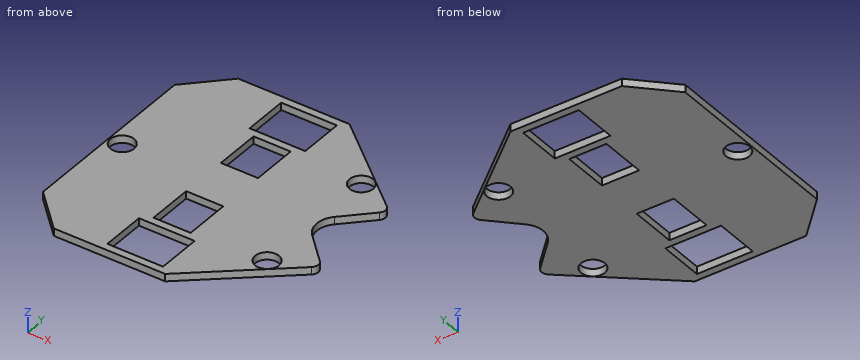
```python
from build123d import *

# Parameters (mm, degrees)
SKETCH_R      = 16
SKETCH_W      = 75
SKETCH_H      = 60
SKETCH_W_2    = 50
SKETCH_H_2    = 62
EXTRUDE_DEPTH = 10


with BuildPart() as part:
    # Sketch → Extrude (new body)
    with BuildSketch(Plane.XY):
        with BuildLine():
            Line((-152.5, 125), (-152.5, -125))
            Line((-152.5, -125), (-102.5, -175))
            Line((-102.5, -175), (47.5, -175))
            Line((47.5, -175), (171.038135, -71.339197))
            ThreePointArc((171.038135, -71.339197), (174.600715, -64.114951), (171.6813, -56.607707))
            Line((136.286797, -21.213204), (171.6813, -56.607707))
            ThreePointArc((136.286797, 21.213204), (127.5, 0), (136.286797, -21.213204))
            Line((171.6813, 56.607707), (136.286797, 21.213204))
            ThreePointArc((171.6813, 56.607707), (174.600715, 64.114951), (171.038135, 71.339197))
            Line((171.038135, 71.339197), (47.5, 175))
            Line((47.5, 175), (-102.5, 175))
            Line((-102.5, 175), (-152.5, 125))
        make_face()
        with Locations((124, 89.5)):
            Circle(SKETCH_R, mode=Mode.SUBTRACT)
        with Locations((124, -89.5)):
            Circle(SKETCH_R, mode=Mode.SUBTRACT)
        with Locations((-134.5, 0)):
            Circle(SKETCH_R, mode=Mode.SUBTRACT)
        with Locations((0, 135)):
            Rectangle(SKETCH_W, SKETCH_H, mode=Mode.SUBTRACT)
        with Locations((0, -135)):
            Rectangle(SKETCH_W, SKETCH_H, mode=Mode.SUBTRACT)
        with Locations((0, 64)):
            Rectangle(SKETCH_W_2, SKETCH_H_2, mode=Mode.SUBTRACT)
        with Locations((0, -64)):
            Rectangle(SKETCH_W_2, SKETCH_H_2, mode=Mode.SUBTRACT)
    extrude(amount=EXTRUDE_DEPTH)


with BuildPart() as part_1:
    # Extrude placement: moved
    add(part.part.moved(Location((0, 0, -30))))


solid = part_1.part
```
The listing builds one solid part. Answer for the finished solid, in the listing's coordinates (mm). Coordinates: 2 decimals unless noted, no trailing zeros. Loops run counter-clockwise (first coordinate to the right, second up) from the corner with the lowest first, then second, coordinate; pieces in that order, holes last. Notation, with made-up numbers: (51.5, 80.5) -> (102.5, 80.5) arc R20 cw to (102.5, 110.5) -> close; hole circle Ø10 at (82.5, 48). An arc over 180 degrees is marked (long way). Return JSON: item names as keys, results as strings. Group by question number.
(1) A cutting plane is placed at B-B on x = -134.5. Write down the section's boundary in (y, z), and give its area (3 significant figures).
(2) Given pin 1 Ø3 at (y, z) = (129.5, -23.5) entering from +X; pin 2 Ø3 at (x, z) = (109.5, -29) entering from +Y; pin 3 Ø2 at (x, z) = (91.5, -24.5) entering from -Y, each flat-ended and moving along its own axis, determine where each tip first touches the part or whether it passes through.
(3) A cutting plane is placed at A-A on z = -25. Count the separate pieces of the cut face and the enclosed holes in it, and give its area (3 significant figures).
(4) A cutting plane is placed at D-D on x = 32. Write down the section's boundary in (y, z).
(5) A cutting plane is placed at C-C on y = 0. Write down the section's boundary in (x, z), and give its area (3 significant figures).
(6) Find the intervals of material crossed by probe 1 along Y at (x, z) = (17.5, -26); probe 2 along Y at (x, z) = (130, -27.5); probe 3 along Y at (x, z) = (124, -23), in increasing order. Write a range as from..to.
The answers:
{
 "1": {"outline": "(-143, -30) -> (-16, -30) -> (-16, -20) -> (-143, -20) -> close; (16, -30) -> (143, -30) -> (143, -20) -> (16, -20) -> close", "area": "2,540 mm^2"},
 "2": {"pin 1": "stops at x = 103.51", "pin 2": "stops at y = 124.23", "pin 3": "stops at y = -138.92"},
 "3": {"separate pieces": "1", "enclosed holes": "7", "area": "77,500 mm^2"},
 "4": {"outline": "(-175, -30) -> (-165, -30) -> (-165, -20) -> (-175, -20) -> close; (-105, -30) -> (105, -30) -> (105, -20) -> (-105, -20) -> close; (165, -30) -> (175, -30) -> (175, -20) -> (165, -20) -> close"},
 "5": {"outline": "(-152.5, -30) -> (-150.5, -30) -> (-150.5, -20) -> (-152.5, -20) -> close; (-118.5, -30) -> (127.5, -30) -> (127.5, -20) -> (-118.5, -20) -> close", "area": "2,480 mm^2"},
 "6": {"probe 1": "y = -175..-165, -105..-95, -33..33, 95..105, 165..175", "probe 2": "y = -105.77..-104.33, -74.67..-11.99, 11.99..74.67, 104.33..105.77", "probe 3": "y = -110.81..-105.5, -73.5..73.5, 105.5..110.81"}
}
